Verification items for the finished model (mm, model axes). Coordinates: 2 decimals unless noted, no trailing zeros. Order: outer loops, then holes, each group sorted by start corner. A loop starts at its lowest first (then second) coordinate and runs counter-clockwise, first axis right, second up. Notation, with made-up numbers: (-30, 24.5) -> (-24, 24.5) arc R19 ccw to (-24, 31.5) -> close; hole circle Ø7 at (-10.75, 74.5). An arc over 180 degrees is marked (long way). Use CSV: the item, a comma, the result in double quotes. Start each with the question number.
1) Sectioned sample at B-B on z = 124. Record the boundary of the cut face in (x, y) (3 decimals), then the cut area to 3 significant figures.
2) Sectioned sample at A-A on x = -124. Record the boundary of the cut face in (y, z) (3 decimals).
3) Go/stop test with flat-tipped pins: pin 1 (1 mm diameter, centred on x = 81.5, z = 44, fed in from -Y); pin 2 (7.5 mm diameter, centred on x = -124, z = 124, fed in from -Y). Record where each tip stops, or that it passes through.
4) Scan lines: line 1 along X through (y, z) = (2.2, 124); line 2 along Z through (x, y) = (-124, 10) (3 decimals); line 3 along X through (y, z) = (10.25, -124) (3 decimals). Record each from-to range of solid material in increasing order.
Autodesk Inventor part; units mm, degrees
ref_plane "YZ Plane" through (0, 0, 0) normal (1, 0, 0) x (0, 1, 0)
ref_plane "XZ Plane" through (0, 0, 0) normal (0, 1, 0) x (-1, 0, 0)
ref_plane "XY Plane" through (0, 0, 0) normal (0, 0, 1) x (1, 0, 0)
sketch "Sketch1" plane through (0, 0, 0) normal (0, 1, 0) x (-1, 0, 0)
  line L0 (-138, 138) -> (138, 138)
  line L1 (138, 138) -> (138, -138)
  line L2 (138, -138) -> (-138, -138)
  line L3 (-138, -138) -> (-138, 138)
  line L4 (-138, 138) -> (138, -138) construction
  line L5 (138, 138) -> (-138, -138) construction
  line L6 (138, 130.5) -> (130.5, 130.5)
  line L7 (130.5, 130.5) -> (130.5, 138)
  point P0 (0, 0)
  dimension "d0" = 276
  dimension "d1" = 276
  dimension "d18" = 7.5
extrude "Extrusion1" add sketch "Sketch1" along normal blind 12
sketch "Sketch3" plane through (0, 12, 0) normal (0, 1, 0) x (1, 0, 0)
  line L0 (-138, 138) -> (-138, -138)
  line L1 (-138, -138) -> (138, -138)
  point P0 (0, 0)
  point P1 (-124, -124)
  dimension "d21" = 14
  dimension "d22" = 14
hole "Hole2" at (-124, 12, 124) direction (0, -1, 0) diameter 7.94 end through all counterbore diameter 9.53 counterbore depth 6
mirror "Mirror1 Right" about plane through (0, 0, 0) normal (0, 0, 1) of "Hole2"
mirror "Mirror2 Bottom" about plane through (0, 0, 0) normal (1, 0, 0) of "Hole2", "Mirror1 Right"
fillet "Fillet1" radius 2 4 edges at (0, 12, 138) (-138, 12, 0) (138, 12, 0) (0, 12, -138)
properties part number "Arrow Panel" material "Polycarbonate, Clear"
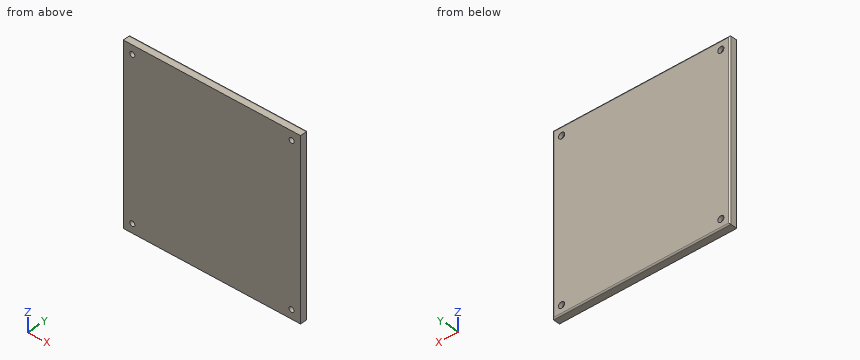
Answers follow:
1,outline,"(-138, 0) -> (-127.97, 0) -> (-127.97, 6) -> (-128.765, 6) -> (-128.765, 12) -> (-136, 12) arc R2 ccw to (-138, 10) -> close; (-120.03, 0) -> (120.03, 0) -> (120.03, 6) -> (119.235, 6) -> (119.235, 12) -> (-119.235, 12) -> (-119.235, 6) -> (-120.03, 6) -> close; (127.97, 0) -> (138, 0) -> (138, 10) arc R2 ccw to (136, 12) -> (128.765, 12) -> (128.765, 6) -> (127.97, 6) -> close"
1,area,"3,100 mm²"
2,outline,"(0, -138) -> (10, -138) arc R2 ccw to (12, -136) -> (12, -128.765) -> (6, -128.765) -> (6, -127.97) -> (0, -127.97) -> close; (0, -120.03) -> (6, -120.03) -> (6, -119.235) -> (12, -119.235) -> (12, 119.235) -> (6, 119.235) -> (6, 120.03) -> (0, 120.03) -> close; (0, 127.97) -> (6, 127.97) -> (6, 128.765) -> (12, 128.765) -> (12, 136) arc R2 ccw to (10, 138) -> (0, 138) -> close"
3,pin 1,"stops at y = 0"
3,pin 2,"passes through"
4,line 1,"x = -138 to -127.97, -120.03 to 120.03, 127.97 to 138"
4,line 2,"z = -138 to -128.765, -119.235 to 119.235, 128.765 to 138"
4,line 3,"x = -137.984 to -128.765, -119.235 to 119.235, 128.765 to 137.984"
